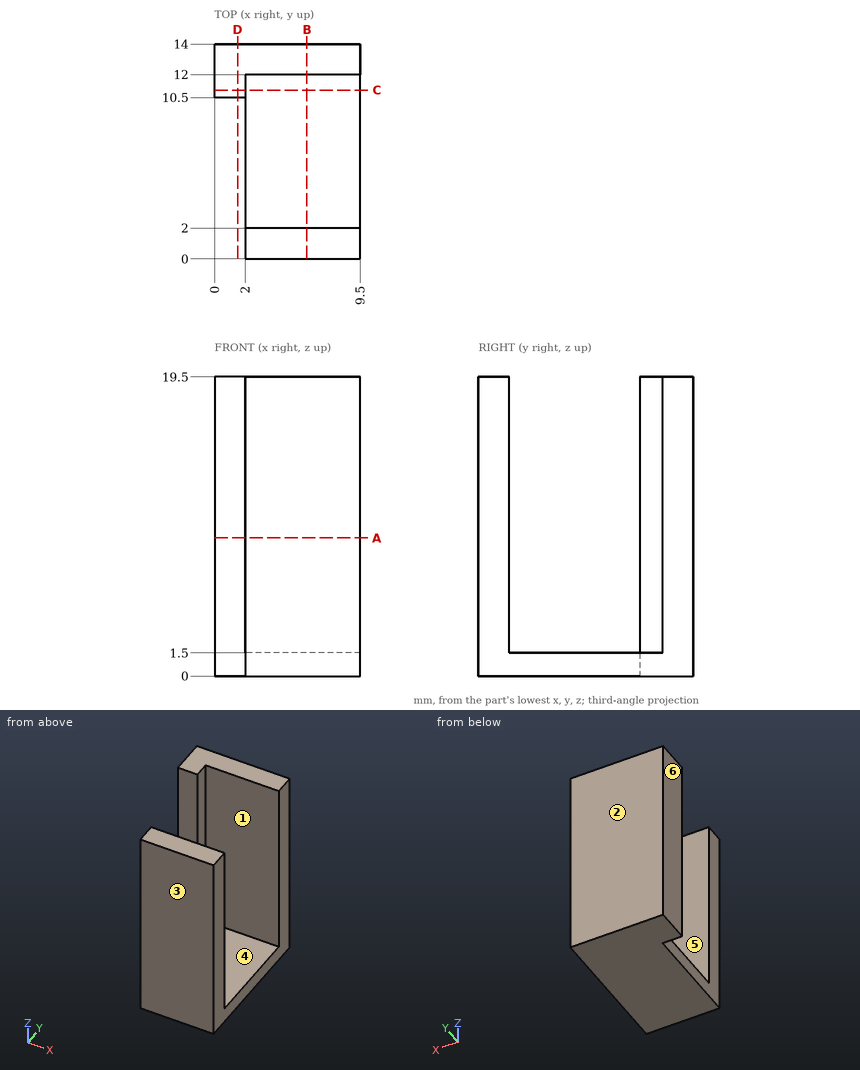
Verification items for this drawing (mm, ordinates from the low corner). A direction names the side the tool comes from. Give positions to 0.01 mm unless a question says otherwise; leave off trailing zeros. Loops run counter-clockwise (first coordinate to the right, second up) from the corner with the lowest first, then second, coordinate; pieces in that order, holes last. Notation, with made-up numbers: M 45,9.25 L 81,9.25 A24 cw 81,42.25 Z; hole C -40,70 d2. An arc over 180 degrees is marked long. Answer in a Markdown table with one row per item.
1) Cross-section at D-D (x = 1.5). Enter the section's corners in (y, z).
Solutions:
| item | result |
|---|---|
| outline | M 10.5,0 L 14,0 L 14,19.5 L 10.5,19.5 Z |
2) Depth check by flat-ended pin: pin 1 (4 mm diameter, centred on x = 6, y = 5, fed in from +Z); pin 2 (1.2 mm diameter, centred on y = 11, z = 9.5, fed in from +X); pin 3 (5 mm diameter, centred on x = 1, y = 12.5, fed in from -Z); pin 4 (1 mm diameter, centred on x = 0.5, z = 8.5, fed in from -Y). Enter the tip coordinate at first touch or a pass-through.
Solutions:
| item | result |
|---|---|
| pin 1 | stops at z = 1.5 |
| pin 2 | stops at x = 2 |
| pin 3 | stops at z = 0 |
| pin 4 | stops at y = 10.5 |
3) Tool access check on the marked faces 5 and 6. Record the directions out of +Z, -Z, +X, -X, +Y, -Y that give a thin tool (end or side, any length) a straight path to the whole face; none if there is none.
Solutions:
| item | result |
|---|---|
| face 5 | +Z, +X, -X |
| face 6 | +Z, -Z, -X, +Y, -Y |
4) Cross-section at B-B (x = 6). Enter the section's corners in (y, z), plus the area to 3 significant figures.
Solutions:
| item | result |
|---|---|
| outline | M 0,0 L 14,0 L 14,19.5 L 12,19.5 L 12,1.5 L 2,1.5 L 2,19.5 L 0,19.5 Z |
| area | 93.0 mm^2 |
5) Cross-section at C-C (y = 11). Enter the section's corners in (x, z), plus the area to 4 significant figures.
Solutions:
| item | result |
|---|---|
| outline | M 0,0 L 9.5,0 L 9.5,1.5 L 2,1.5 L 2,19.5 L 0,19.5 Z |
| area | 50.25 mm^2 |
6) Mould release check, pull along Y, two halves, no side actions. Record for the marked faces 1, 2, 3 and 4: released by +Y, released by -Y, zero draft, split by the parting line, or undercut.
Solutions:
| item | result |
|---|---|
| face 1 | undercut |
| face 2 | released by +Y |
| face 3 | released by -Y |
| face 4 | undercut |
7) Thickness scan on line 1 (Y direction, x = 8.75, z = 8.25); line 2 (Z direction, x = 3.75, y = 3); line 3 (Y direction, x = 1.25, z = 14.5). Record the ranges inside material, lowest first.
Solutions:
| item | result |
|---|---|
| line 1 | y = 0 to 2, 12 to 14 |
| line 2 | z = 0 to 1.5 |
| line 3 | y = 10.5 to 14 |
8) Cross-section at A-A (z = 9). Enter the section's corners in (x, y), plus the area to 3 significant figures.
Solutions:
| item | result |
|---|---|
| outline | M 0,10.5 L 2,10.5 L 2,12 L 9.5,12 L 9.5,14 L 0,14 Z; M 2,0 L 9.5,0 L 9.5,2 L 2,2 Z |
| area | 37.0 mm^2 |
